from build123d import *

# Parameters (mm, degrees)
SKETCH_R             = 2.95
PAD_DEPTH            = 1.8
SKETCH_MIRRORED_2_R  = 2.95
PAD_MIRRORED_2_DEPTH = 1.8


with BuildPart() as part:
    # Sketch → Pad (new body)
    with BuildSketch(Plane.XY):
        with BuildLine():
            Line((0, 0), (30, 0))
            Line((30, 0), (30, 61))
            ThreePointArc((30, 61), (29.12132, 63.12132), (27, 64))
            Line((27, 64), (0, 64))
            Line((0, 64), (0, 0))
        make_face()
        with Locations((25, 59)):
            Circle(SKETCH_R, mode=Mode.SUBTRACT)
    pad = extrude(amount=PAD_DEPTH)

    # Sketch Mirrored 2 → Pad Mirrored 2 (add)
    with BuildSketch(Plane(origin=(0, 0, 0), x_dir=(-1, 0, 0), z_dir=(0, 0, -1))):
        with BuildLine():
            Line((0, 0), (30, 0))
            Line((30, 0), (30, 61))
            ThreePointArc((30, 61), (29.12132, 63.12132), (27, 64))
            Line((27, 64), (0, 64))
            Line((0, 64), (0, 0))
        make_face()
        with Locations((25, 59)):
            Circle(SKETCH_MIRRORED_2_R, mode=Mode.SUBTRACT)
    pad_mirrored_2 = extrude(amount=-PAD_MIRRORED_2_DEPTH)

    # Mirrored001: Pad, Pad Mirrored 2 across Sketch H_Axis
    add(pad.mirror(Plane.ZX))
    add(pad_mirrored_2.mirror(Plane.ZX))


solid = part.part
Input: part model. Units: mm. Frame: model coordinates. Give positions to 0.01 mm unless a question says otherwise; leave off trailing zeros. Write each loop counter-clockwise with the first axis right and the second up, starting at its lowest first coordinate (ties: lowest second). Pieces come first, ordered by that corner, then holes.
Q1. Section A-A, the plane y = 59. Output: boundary loops of the cut face in (x, z), plus the area to 3 significant figures.
Q2. Material intervals for probe 1 along Y at (x, z) = (-25, 0.6); probe 2 along X at (y, z) = (-59, 0.6); probe 3 along X at (y, z) = (-57.5, 0.8), sorted ascending.
Q3. Section C-C, the plane x = -25. Output: boundary loops of the cut face in (y, z).
Q4. Pull-direction query (Y, two-part tool) for faces 1 (the face through (29.14, 63.1, 0.89)), 2 (the face through (29.14, -63.1, 0.89)), 3 (the face through (-26.36, -56.38, 0.89)), 4 (the face through (0, -1, 0)); classes: pulls with the +Y half, pulls with the -Y half, needs draft (parallel to the pull), parting line crosses it, or undercut.
Q5. Section B-B, the plane z = 0.9. Output: boundary loops of the cut face in (x, y).
Filled in:
1. outline: (-30, 0) - (-27.95, 0) - (-27.95, 1.8) - (-30, 1.8) - close; (-22.05, 0) - (22.05, 0) - (22.05, 1.8) - (-22.05, 1.8) - close; (27.95, 0) - (30, 0) - (30, 1.8) - (27.95, 1.8) - close
1. area: 86.8 mm2
2. probe 1: y = -64 to -61.95, -56.05 to 56.05, 61.95 to 64
2. probe 2: x = -30 to -27.95, -22.05 to 22.05, 27.95 to 30
2. probe 3: x = -30 to -27.54, -22.46 to 22.46, 27.54 to 30
3. outline: (-64, 0) - (-61.95, 0) - (-61.95, 1.8) - (-64, 1.8) - close; (-56.05, 0) - (56.05, 0) - (56.05, 1.8) - (-56.05, 1.8) - close; (61.95, 0) - (64, 0) - (64, 1.8) - (61.95, 1.8) - close
4. face 1: pulls with the +Y half
4. face 2: pulls with the -Y half
4. face 3: undercut
4. face 4: needs draft
5. outline: (-30, -61) arc R3 ccw to (-27, -64) - (27, -64) arc R3 ccw to (30, -61) - (30, 61) arc R3 ccw to (27, 64) - (-27, 64) arc R3 ccw to (-30, 61) - close; hole circle Ø5.9 at (-25, -59); hole circle Ø5.9 at (-25, 59); hole circle Ø5.9 at (25, -59); hole circle Ø5.9 at (25, 59)
